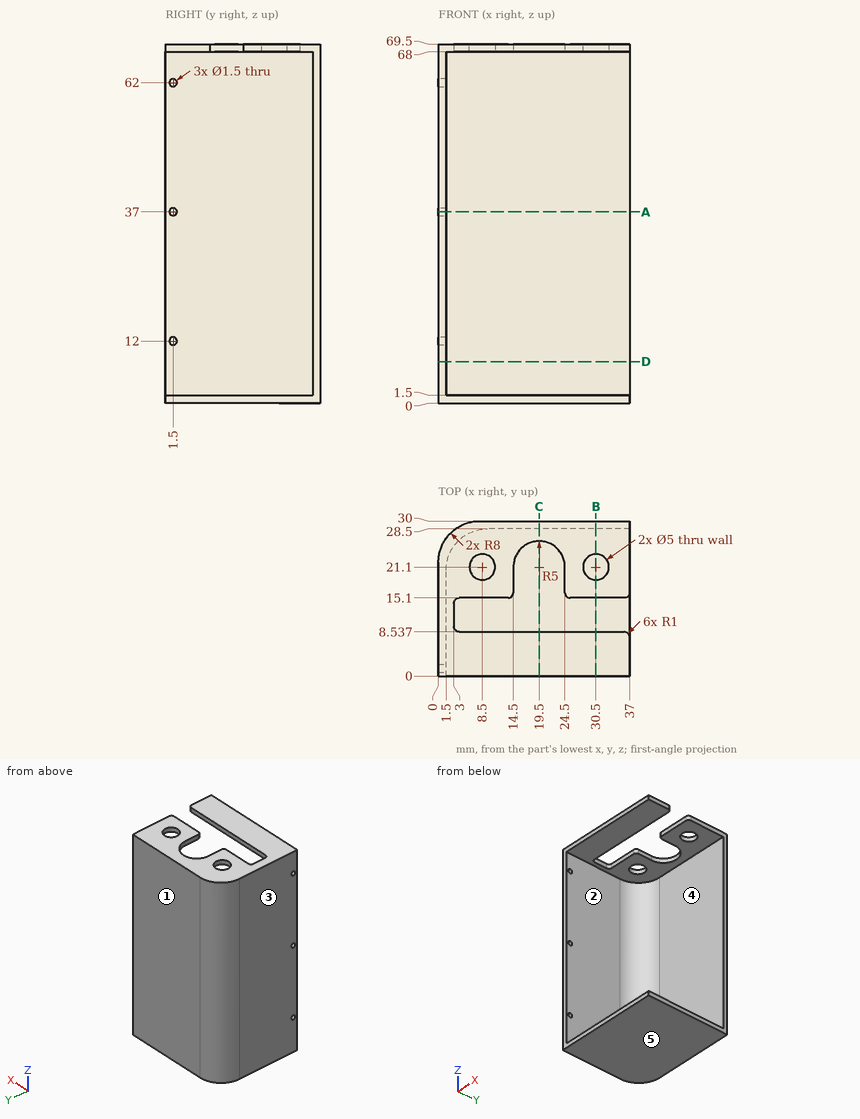
Geometry check sheet. Reference: drawing and pictorial views, mm from the part's lowest x, y, z. A direction names the side the tool comes from. Coordinates: 2 decimals unless noted, no trailing zeros. Order: outer loops, then holes, each group sorted by start corner. A loop starts at its lowest first (then second) coordinate and runs counter-clockwise, first axis right, second up.
Item 1: Depth check by flat-ended pin: pin 1 (22 mm diameter, centred on x = 27, z = 48, fed in from -Y); pin 2 (6 mm diameter, centred on y = 6.5, z = 34.5, fed in from +X); pin 3 (1.5 mm diameter, centred on y = 23.5, z = 41, fed in from -X) (1 decimal). Enter the tip coordinate at first touch or a pass-through.
Item 2: Tool access check on the marked faces 1 and 2. Record the directions out of +Z, -Z, +X, -X, +Y, -Y that give a thin tool (end or side, any length) a straight path to the whole face; none if there is none.
Item 3: Section check C-C (x = 19.5). Enter the section's corners in (y, z).
Item 4: Section check B-B (x = 30.5). Enter the section's corners in (y, z).
Item 5: Section check A-A (z = 37). Enter the section's corners in (x, y), plus the area to 3 significant figures.
Item 6: Mould release check, pull along Z, two halves, no side actions. Record for the marked faces 3, 4 and 5: released by +Z, released by -Z, zero draft, split by the parting line, or undercut.
Item 7: Section check D-D (z = 8). Enter the section's corners in (x, y).
Item 8: Scan lines: line 1 along Y through (x, z) = (30.5, 68.75); line 2 along Z through (x, y) = (16, 2); line 3 along Z through (x, y) = (0.7, 1.5). Record each from-to range of solid material in increasing order.
Check sheet entries:
1. pin 1: stops at y = 28.5
1. pin 2: stops at x = 1.5
1. pin 3: stops at x = 0
2. face 1: +Z, -Z, +X, -X, +Y
2. face 2: +X, -Y
3. outline: (0, 0) - (30, 0) - (30, 69.5) - (26.1, 69.5) - (26.1, 68) - (28.5, 68) - (28.5, 1.5) - (0, 1.5) - close; (0, 68) - (8.54, 68) - (8.54, 69.5) - (0, 69.5) - close
4. outline: (0, 0) - (30, 0) - (30, 69.5) - (23.6, 69.5) - (23.6, 68) - (28.5, 68) - (28.5, 1.5) - (0, 1.5) - close; (0, 68) - (8.54, 68) - (8.54, 69.5) - (0, 69.5) - close; (15.1, 68) - (18.6, 68) - (18.6, 69.5) - (15.1, 69.5) - close
5. outline: (0, 0) - (1.5, 0) - (1.5, 0.75) - (0, 0.75) - close; (0, 2.25) - (1.5, 2.25) - (1.5, 20.5) arc R8 cw to (9.5, 28.5) - (37, 28.5) - (37, 30) - (8, 30) arc R8 ccw to (0, 22) - close
5. area: 96.0 mm2
6. face 3: zero draft
6. face 4: undercut
6. face 5: released by -Z
7. outline: (0, 0) - (1.5, 0) - (1.5, 20.5) arc R8 cw to (9.5, 28.5) - (37, 28.5) - (37, 30) - (8, 30) arc R8 ccw to (0, 22) - close
8. line 1: y = 0 to 8.54, 15.1 to 18.6, 23.6 to 30
8. line 2: z = 0 to 1.5, 68 to 69.5
8. line 3: z = 0 to 11.25, 12.75 to 36.25, 37.75 to 61.25, 62.75 to 69.5
